Input: part model. Units: mm. Frame: model coordinates. A direction names the side the tool comes from. Round coordinates to 2 decimals unless told otherwise and drop trailing zeros. Order: outer loops, then holes, each group sorted by start corner. A loop starts at its lowest first (then second) coordinate and runs counter-clockwise, first axis right, second up. Notation, with made-up numbers: (60.5, 3.25) - (99.5, 3.25) arc R13 ccw to (99.5, 8.25) - close; hole circle Ø3 at (-9.5, 65.5). An arc over 180 degrees is marked (long way). One line per item, written item: value. Start each with the question number.
from build123d import *

# Parameters (mm, degrees)
SKETCH_2_R          = 73.899050909
EXTRUDE_2_DEPTH     = 3
SKETCH_6_OUTSIDE_W  = 191.606
SKETCH_6_OUTSIDE_H  = 191.606
CUT_EXTRUDE_4_DEPTH = 10
SKETCH_7_R          = 4.5
SKETCH_7_R_2        = 2
CUT_EXTRUDE_5_DEPTH = 10
SKETCH_8_R          = 4.5
CUT_EXTRUDE_6_DEPTH = 10
SKETCH_9_W          = 6.25
SKETCH_9_H          = 33
SKETCH_9_R          = 2
EXTRUDE_3_DEPTH     = 20
SKETCH_10_W         = 6.25
SKETCH_10_H         = 30
CUT_EXTRUDE_7_DEPTH = 17
SKETCH_11_W         = 1.5
SKETCH_11_H         = 33
SKETCH_11_W_2       = 1.098612182
EXTRUDE_4_DEPTH     = 2.999995
FILLET_1_R          = 3


with BuildPart() as part:
    # 草图2 → 凸台-拉伸2 (new body)
    with BuildSketch(Plane.XY):
        Circle(SKETCH_2_R)
    extrude(amount=EXTRUDE_2_DEPTH)

    # 草图6 outside → 切除-拉伸4 (cut)
    with BuildSketch(Plane.XY.offset(3)):
        Rectangle(SKETCH_6_OUTSIDE_W, SKETCH_6_OUTSIDE_H)
        with BuildLine():
            Line((-31.535008434, 35.392907634), (-24.330725879, 30.255179498))
            ThreePointArc((-24.330725879, 30.255179498), (-24.094123176, 29.977447186), (-24.016566775, 29.6209348))
            Line((-24.016566775, 29.6209348), (-24.048055472, 28.621430692))
            ThreePointArc((-24.048055472, 28.621430692), (-23.970499071, 28.264918306), (-23.733896368, 27.987185994))
            Line((-23.733896368, 27.987185994), (-14.617442117, 21.485794197))
            ThreePointArc((-14.617442117, 21.485794197), (-14.277785331, 21.352567532), (-13.915454513, 21.395374713))
            Line((-13.915454513, 21.395374713), (-12.980724299, 21.750732881))
            ThreePointArc((-12.980724299, 21.750732881), (-12.618393481, 21.793540061), (-12.278736695, 21.660313397))
            ThreePointArc((-12.278736695, 21.660313397), (-3.294948021, 19.590594088), (4.517495731, 24.485276874))
            ThreePointArc((4.517495731, 24.485276874), (4.794882728, 24.722284322), (5.15128164, 24.800360515))
            Line((5.15128164, 24.800360515), (6.150830603, 24.770329354))
            ThreePointArc((6.150830603, 24.770329354), (6.507229515, 24.848405547), (6.784616512, 25.085412994))
            Line((6.784616512, 25.085412994), (13.272707556, 34.211338045))
            ThreePointArc((13.272707556, 34.211338045), (13.405438783, 34.551188744), (13.362103288, 34.913456755))
            Line((13.362103288, 34.913456755), (13.005382451, 35.847667782))
            ThreePointArc((13.005382451, 35.847667782), (12.962046956, 36.209935793), (13.094778183, 36.549786492))
            Line((13.094778183, 36.549786492), (18.221995392, 43.761553351))
            ThreePointArc((18.221995392, 43.761553351), (18.708323153, 44.066496264), (19.267836012, 43.938237808))
            Line((19.267836012, 43.938237808), (23.750427961, 40.751331876))
            ThreePointArc((23.750427961, 40.751331876), (24.055370874, 40.265004115), (23.927112418, 39.705491256))
            ThreePointArc((23.927112418, 39.705491256), (23.798853962, 39.145978396), (24.103796875, 38.659650636))
            Line((24.103796875, 38.659650636), (31.031438978, 33.734432377))
            ThreePointArc((31.031438978, 33.734432377), (31.336381891, 33.248104616), (31.208123435, 32.688591757))
            Line((31.208123435, 32.688591757), (27.586639421, 27.59473727))
            Line((27.586639421, 27.59473727), (29.886186599, 21.936685188))
            ThreePointArc((29.886186599, 21.936685188), (29.936337177, 21.567492307), (29.80264047, 21.219722765))
            Line((29.80264047, 21.219722765), (24.485385754, 13.740655704))
            ThreePointArc((24.485385754, 13.740655704), (24.200836556, 13.500134983), (23.835658301, 13.426220802))
            Line((23.835658301, 13.426220802), (17.736202905, 13.739453063))
            Line((17.736202905, 13.739453063), (14.114718892, 8.645598576))
            ThreePointArc((14.114718892, 8.645598576), (13.628391131, 8.340655663), (13.068878271, 8.468914119))
            Line((13.068878271, 8.468914119), (9.306333892, 11.143901076))
            Line((9.306333892, 11.143901076), (15.851133659, -27.769160612))
            ThreePointArc((15.851133659, -27.769160612), (6.806822505, -40.470956104), (-5.894972987, -31.42664495))
            Line((-5.894972987, -31.42664495), (-12.439772753, 7.486416738))
            Line((-12.439772753, 7.486416738), (-15.120243503, 3.727777092))
            ThreePointArc((-15.120243503, 3.727777092), (-15.607015422, 3.423543678), (-16.166340657, 3.552617894))
            Line((-16.166340657, 3.552617894), (-21.25490879, 7.181526042))
            Line((-21.25490879, 7.181526042), (-26.916308113, 4.890232022))
            ThreePointArc((-26.916308113, 4.890232022), (-27.285573732, 4.840619864), (-27.633147944, 4.974823555))
            Line((-27.633147944, 4.974823555), (-35.1044533, 10.30297878))
            ThreePointArc((-35.1044533, 10.30297878), (-35.344558829, 10.587878409), (-35.41794042, 10.953164059))
            Line((-35.41794042, 10.953164059), (-35.095814113, 17.052156207))
            Line((-35.095814113, 17.052156207), (-40.184382246, 20.681064356))
            ThreePointArc((-40.184382246, 20.681064356), (-40.48861566, 21.167836275), (-40.359541444, 21.727161509))
            Line((-40.359541444, 21.727161509), (-35.424226362, 28.647614171))
            ThreePointArc((-35.424226362, 28.647614171), (-35.295152147, 29.206939406), (-35.59938556, 29.693711325))
            ThreePointArc((-35.59938556, 29.693711325), (-35.903618974, 30.180483244), (-35.774544759, 30.739808479))
            Line((-35.774544759, 30.739808479), (-32.581105588, 35.217748436))
            ThreePointArc((-32.581105588, 35.217748436), (-32.094333668, 35.521981849), (-31.535008434, 35.392907634))
        make_face(mode=Mode.SUBTRACT)
    extrude(amount=-CUT_EXTRUDE_4_DEPTH, mode=Mode.SUBTRACT)

    # 草图7 → 切除-拉伸5 (cut)
    with BuildSketch(Plane.XY.offset(3)):
        with Locations((4.978080336, -29.597902781)):
            Circle(SKETCH_7_R)
        with Locations((3.651194467, -21.708709293)):
            Circle(SKETCH_7_R_2)
        with Locations((12.867273824, -28.271016911)):
            Circle(SKETCH_7_R_2)
        with Locations((6.304966206, -37.487096269)):
            Circle(SKETCH_7_R_2)
        with Locations((-2.911113152, -30.924788651)):
            Circle(SKETCH_7_R_2)
    extrude(amount=-CUT_EXTRUDE_5_DEPTH, mode=Mode.SUBTRACT)

    # 草图8 → 切除-拉伸6 (cut)
    with BuildSketch(Plane.XY.offset(3)):
        with Locations((-24.401296977, 17.408951983)):
            Circle(SKETCH_8_R)
        with Locations((17.442589177, 24.41531991)):
            Circle(SKETCH_8_R)
    extrude(amount=-CUT_EXTRUDE_6_DEPTH, mode=Mode.SUBTRACT)

    # 镜向3: part across plane


with BuildPart() as part_1:
    add(part.part)
    add(part.part.mirror(Plane(origin=(0, 0, 0), x_dir=(0, 0, 1), z_dir=(-0.9861491859840638, -0.16586073369839163, 0))))

    # 草图9 → 凸台-拉伸3 (add)
    with BuildSketch(Plane(origin=(-3.770666854, -5.287346609, 0), x_dir=(0.814170901346189, -0.5806253037899178, 0), z_dir=(-0.5806253037899178, -0.814170901346189, 0))):
        with Locations((-41.599903988, -13.5)):
            Rectangle(SKETCH_9_W, SKETCH_9_H)
        with Locations(Location((-41.452827346, -24, 0), (0, 0, 180))):
            Circle(SKETCH_9_R, mode=Mode.SUBTRACT)
        with Locations(Location((-41.452827346, -6, 0), (0, 0, 180))):
            Circle(SKETCH_9_R, mode=Mode.SUBTRACT)
    extrude(amount=-EXTRUDE_3_DEPTH)

    # 草图10 → 切除-拉伸7 (cut)
    with BuildSketch(Plane(origin=(-3.770666854, -5.287346609, 0), x_dir=(0.8141709013461893, -0.5806253037899172, 0), z_dir=(-0.5806253037899172, -0.8141709013461893, 0))):
        with Locations((-41.599903988, -15)):
            Rectangle(SKETCH_10_W, SKETCH_10_H)
    extrude(amount=-CUT_EXTRUDE_7_DEPTH, mode=Mode.SUBTRACT)

    # 草图11 → 凸台-拉伸4 (add)
    with BuildSketch(Plane(origin=(6.09996331, 8.553558714, 0), x_dir=(0.8141709013461892, -0.5806253037899176, 0), z_dir=(0.5806253037899175, 0.8141709013461891, 0))):
        with Locations((-45.474903988, 13.5)):
            Rectangle(SKETCH_11_W, SKETCH_11_H)
        with Locations((-37.925597897, 13.5)):
            Rectangle(SKETCH_11_W_2, SKETCH_11_H)
    extrude(amount=EXTRUDE_4_DEPTH)

    # 圆角1
    fillet_1_edges = [part_1.edges().sort_by_distance(p)[0] for p in [
        (-31.535008434, 35.392907634, 1.5),
        (-24.330725879, 30.255179498, 1.5),
        (-23.459789375, 31.476433815, -30),
        (-30.66407193, 36.614161951, -30),
    ]]
    fillet(fillet_1_edges, radius=FILLET_1_R)

    # 镜向4: part across plane


with BuildPart() as part_2:
    add(part_1.part)
    add(part_1.part.mirror(Plane(origin=(0, 0, 0), x_dir=(0, 0, 1), z_dir=(-0.9861491859840638, -0.16586073369839163, 0))))


solid = part_2.part
Item 1: Section query B-B on y = 15. Return loops of the section in (x, z), and give its area (3 significant figures).
Item 2: First-contact query: pin 1 Ø11.5 at (x, y) = (4.98, -29.6) entering from -Z. Flat tip, straight axial feed; report the tip coordinate or a pass-through.
Item 3: Pull-direction query (Y, two-part tool) for faces 5 (the face through (-24.182, 32.017, -29.145)), 6 (the face through (13.122, 41.766, -13.269)), 7 (the face through (-28.27, 15.11, 1.52)); classes: released by +Y, released by -Y, zero draft, split by the parting line, or undercut.
Item 4: Reachability of faces 1 (the face through (-27.98, 32.86, -15.21)), 2 (the face through (12.378, 38.166, -29.145)), 3 (the face through (15.694, 40.206, -15.21)), 4 (the face through (-30.676, 36.597, -11.79)) from +Z, -Z, +X, -X, +Y, -Y: full face, straight path, thin tool, end or side. Return the list, or none.
Item 5: Line query: L1, parallel to Z at x = 14.5, y = -24; L2, parallel to X at y = -23.5, z = 1; L3, parallel to X at y = 37.5, z = -10. Output: solid intervals per line, ascending.
Item 6: Section query C-C on z = -5. Give the number of separate pieces and of enclosed holes in the cut face, and give its area (3 significant figures).
Item 7: Section query D-D on y = 1. Return loops of the section in (x, z), and give its area (3 significant figures).
Geometry results:
1. outline: (-35.2, 0) - (-28.2, 0) - (-28.2, 3) - (-35.2, 3) - close; (-20.64, 0) - (25.38, 0) - (25.38, 3) - (-20.64, 3) - close
1. area: 159 mm^2
2. pin 1: stops at z = 0
3. face 5: released by -Y
3. face 6: released by +Y
3. face 7: undercut
4. face 1: -Z, -X, -Y
4. face 2: -Z, -Y
4. face 3: -Z, +X, -Y
4. face 4: -Z, -X, +Y
5. L1: z = 0 to 3
5. L2: x = -7.23 to 2.76, 4.54 to 15.13
5. L3: x = -30.03 to -29.32, 11.76 to 13.77
6. separate pieces: 4
6. enclosed holes: 0
6. area: 32.3 mm^2
7. outline: (-11.35, 0) - (11.01, 0) - (11.01, 3) - (-11.35, 3) - close
7. area: 67.1 mm^2
